CAD build for the part. Positions are in the model's coordinates, mm. Face numbers are marked on the shaded views. A direction names the side the tool comes from. Round coordinates to 2 decimals unless told otherwise and drop trailing zeros. Write each loop counter-clockwise with the first axis right and the second up, starting at its lowest first coordinate (ties: lowest second). Pieces come first, ordered by that corner, then holes. Notation, with made-up numbers: (-2, 22.25) - (33, 22.25) arc R20 ccw to (33, 41.25) - close; hole circle Ø11 at (23, 87). An arc over 180 degrees is marked (long way). Answer in a Markdown table with one row per item.
```python
from build123d import *

# Parameters (mm, degrees)
SKETCH_1_W          = 60
SKETCH_1_H          = 45
EXTRUDE_2_DEPTH     = 54
SKETCH_4_W          = 55
SKETCH_4_H          = 40
CUT_EXTRUDE_3_DEPTH = 54
SKETCH_5_R          = 2.25
CUT_EXTRUDE_4_DEPTH = 27
SKETCH_6_R          = 2.1
CUT_EXTRUDE_5_DEPTH = 27
EXTRUDE_3_DEPTH     = 54


with BuildPart() as part:
    # 草图1 → 凸台-拉伸2 (new body)
    with BuildSketch(Plane(origin=(0, 0, 0), x_dir=(0, 0, -1), z_dir=(1, 0, 0))):
        with Locations((28.844429728, 4.579365776)):
            Rectangle(SKETCH_1_W, SKETCH_1_H)
    extrude(amount=EXTRUDE_2_DEPTH)

    # 草图4 → 切除-拉伸3 (cut)
    with BuildSketch(Plane(origin=(54, 0, 0), x_dir=(0, 0, -1), z_dir=(1, 0, 0))):
        with Locations((31.344429728, 7.079365776)):
            Rectangle(SKETCH_4_W, SKETCH_4_H)
    extrude(amount=-CUT_EXTRUDE_3_DEPTH, mode=Mode.SUBTRACT)

    # 草图5 → 切除-拉伸4 (cut, symmetric)
    with BuildSketch(Plane(origin=(0, 0, -3.844429728), x_dir=(-1, 0, 0), z_dir=(0, 0, -1))):
        with Locations(Location((-42, 17.653246287, 0), (0, 0, 180))):
            Circle(SKETCH_5_R)
        with Locations(Location((-12, 17.653246287, 0), (0, 0, 180))):
            Circle(SKETCH_5_R)
    extrude(amount=CUT_EXTRUDE_4_DEPTH, both=True, mode=Mode.SUBTRACT)

    # 草图6 → 切除-拉伸5 (cut, symmetric)
    with BuildSketch(Plane(origin=(0, -12.920634224, 0), x_dir=(1, 0, 0), z_dir=(0, 1, 0))):
        with Locations(Location((11, 48.844429728, 0), (0, 0, 270))):
            Circle(SKETCH_6_R)
        with Locations(Location((41, 48.844429728, 0), (0, 0, 270))):
            Circle(SKETCH_6_R)
        with Locations(Location((11, 18.844429728, 0), (0, 0, 270))):
            Circle(SKETCH_6_R)
        with Locations(Location((41, 18.844429728, 0), (0, 0, 270))):
            Circle(SKETCH_6_R)
    extrude(amount=CUT_EXTRUDE_5_DEPTH, both=True, mode=Mode.SUBTRACT)

    # 草图7 → 凸台-拉伸3 (add)
    with BuildSketch(Plane(origin=(54, 0, 0), x_dir=(0, 0, -1), z_dir=(1, 0, 0))):
        Polygon((3.844429728, -2.920634224), (8.844429728, -12.920634224), (3.844429728, -12.920634224), align=None)
    extrude(amount=-EXTRUDE_3_DEPTH)


solid = part.part
```
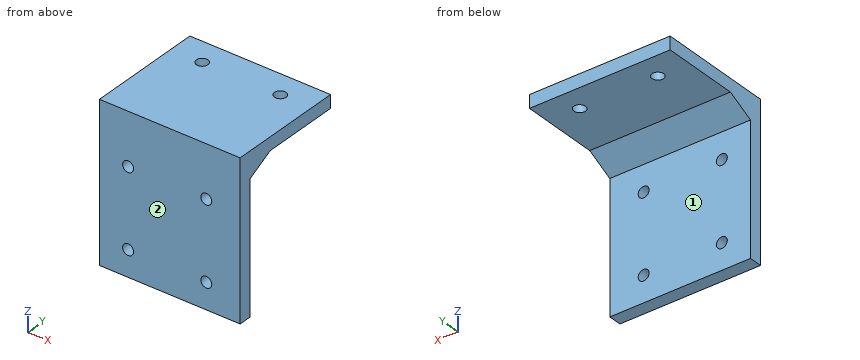
Q1. Saw through at D-D on z = -30. List the corners of the cut face in (x, y).
Computed:
| item | result |
|---|---|
| outline | (0, -17.92) - (54, -17.92) - (54, -12.92) - (0, -12.92) - close |
Q2. 3-axis set-ups, long thin cutter, end or side, ignore diameter. For the marked faces 1 and 2: which of +Z, -Z, +X, -X, +Y, -Y reach the whole face in a straight line?
Computed:
| item | result |
|---|---|
| face 1 | -Z, +X, -X, +Y |
| face 2 | +Z, -Z, +X, -X, -Y |
Q3. Drill centre lines: line 1 (Y direction, x = 12, z = -0.3); line 2 (Z direction, x = 47.5, y = 15); line 3 (Y direction, x = 9, z = -32). Where is each one in solid material? Low to high.
Computed:
| item | result |
|---|---|
| line 1 | y = -17.92 to 15.4, 19.9 to 27.08 |
| line 2 | z = -3.84 to 1.16 |
| line 3 | y = -17.92 to -12.92 |
Q4. Saw through at C-C on y = 8.5. List the corners of the cut face in (x, z).
Computed:
| item | result |
|---|---|
| outline | (0, -3.84) - (54, -3.84) - (54, 1.16) - (0, 1.16) - close |
Q5. Saw through at A-A on x = 30.5. List the corners of the cut face in (y, z), then the cut area to 3 significant figures.
Computed:
| item | result |
|---|---|
| outline | (-17.92, -58.84) - (-12.92, -58.84) - (-12.92, -8.84) - (-2.92, -3.84) - (27.08, -3.84) - (27.08, 1.16) - (-17.92, 1.16) - close |
| area | 525 mm2 |
Q6. Saw through at B-B on x = 11. List the corners of the cut face in (y, z), then the cut area to 3 significant figures.
Computed:
| item | result |
|---|---|
| outline | (-17.92, -58.84) - (-12.92, -58.84) - (-12.92, -50.94) - (-17.92, -50.94) - close; (-17.92, -46.74) - (-12.92, -46.74) - (-12.92, -20.94) - (-17.92, -20.94) - close; (-17.92, -16.74) - (-12.92, -16.74) - (-12.92, -8.84) - (-2.92, -3.84) - (15.64, -3.84) - (15.64, 1.16) - (-17.92, 1.16) - close; (19.67, -3.84) - (27.08, -3.84) - (27.08, 1.16) - (19.67, 1.16) - close |
| area | 463 mm2 |
Q7. Flat gauge pins, fed straight in: pin 1 (3.5 mm diameter, centred on x = 11, z = -18.84, fed in from -Y); pin 2 (6 mm diameter, centred on x = 12, y = 17.65, fed in from +Z); pin 3 (4 mm diameter, centred on x = 9.5, z = -38, fed in from +Y); pin 4 (24 mm diameter, centred on x = 24.5, y = 14.5, fed in from -Z). Where does each tip first touch, or does it go through?
Computed:
| item | result |
|---|---|
| pin 1 | passes through |
| pin 2 | stops at z = 1.16 |
| pin 3 | stops at y = -12.92 |
| pin 4 | stops at z = -3.84 |
